Check sheet for the modelled part. Datum: model origin and axes. Units: mm. Face numbers are marked on the shaded views. A direction names the side the tool comes from. Give positions to 0.01 mm unless a question says otherwise; leave off trailing zeros. Loops run counter-clockwise (first coordinate to the right, second up) from the corner with the lowest first, then second, coordinate; pieces in that order, holes last. Notation, with made-up numbers: M 89.25,68 L 142.25,68 A24 cw 142.25,88 Z; hole C 67.25,-0.75 d3. An arc over 180 degrees is marked long. One line per question, with ' | ' between items. Start each with the question number.
from build123d import *

# Parameters (mm, degrees)
SKETCH3_W          = 10.3
SKETCH3_H          = 10.3
CUT_EXTRUDE1_DEPTH = 10.4
SKETCH4_R          = 2.15
CUT_EXTRUDE2_DEPTH = 16.780339887
CUT_EXTRUDE3_START = -10
SKETCH5_R          = 4.5
CUT_EXTRUDE3_DEPTH = 6.62545693
CHAMFER1_SIZE      = 0.5
CHAMFER1_SIZE2     = 1.37373871


with BuildPart() as part:
    # Sketch2 → Revolve1 (revolve)
    with BuildSketch(Plane(origin=(0, 0, 0), x_dir=(1, 0, 0), z_dir=(0, 1, 0))):
        with BuildLine():
            Line((0, 15), (0, -11.180339887))
            Line((0, -11.180339887), (10, -11.180339887))
            ThreePointArc((10, -11.180339887), (14.012585384, 5.352331347), (0, 15))
        make_face()
    revolve(axis=Axis((0, 0, 15), (0, 0, -1)))

    # Sketch3 → Cut-Extrude1 (cut)
    with BuildSketch(Plane.XY.offset(11.180339887)):
        Rectangle(SKETCH3_W, SKETCH3_H)
    extrude(amount=-CUT_EXTRUDE1_DEPTH, mode=Mode.SUBTRACT)

    # Sketch4 → Cut-Extrude2 (cut, through all)
    with BuildSketch(Plane.XY.offset(0.780339887)):
        Circle(SKETCH4_R)
    extrude(amount=-CUT_EXTRUDE2_DEPTH, mode=Mode.SUBTRACT)

    # Sketch5 → Cut-Extrude3 (cut, through all)
    with BuildSketch(Plane.XY.offset(0.780339887).offset(CUT_EXTRUDE3_START)):
        Circle(SKETCH5_R)
    extrude(amount=-CUT_EXTRUDE3_DEPTH, mode=Mode.SUBTRACT)

    # Chamfer1
    chamfer1_edges = [part.edges().sort_by_distance(p)[0] for p in [
        (5.15, 0, 11.180339887),
        (0, 5.15, 11.180339887),
        (-5.15, 0, 11.180339887),
        (0, -5.15, 11.180339887),
    ]]
    chamfer1_side = [part.faces().sort_by_distance(p)[0] for p in [
        (-9.717157288, 0, 11.180339887),
    ]]
    chamfer(chamfer1_edges, length=CHAMFER1_SIZE, length2=CHAMFER1_SIZE2, reference=chamfer1_side[0])


solid = part.part
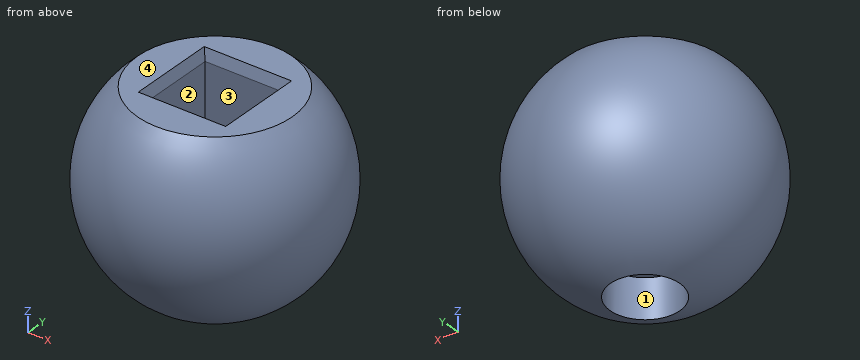
Q1. Material ranges on probe 1 along X at (y, z) = (-0.5, -3.75); probe 2 along Z at (x, y) = (-2.75, -0.25); probe 3 along X at (y, z) = (0, -10.75), recorded low to high. Write a range as from..to.
Q2. Access from +Z, -Z, +X, -X, +Y, -Y to the whole of each face (thin tool, end or side, straight path). Record for the marked faces 1 and 2.
Q3. Cross-section at C-C (z = 8.25). Record the cut outline in (x, y), and give its area (3 significant figures).
Q4. Depth check by flat-ended pin: P1, Ø3, axis at x = 7.5, z = -1.5, coming from the -Y side; P2, Ø4.5, axis at x = 0.5, z = 4.5, coming from the +Y side; P3, Ø11.5, axis at x = -2.5, y = 1, coming from the +Z side; P4, Ø4.5, axis at x = 0, z = 7, coming from the -Y side. Enter the tip coordinate at first touch or a pass-through.
Q5. Cross-section at D-D (z = -8). Record the cut outline in (x, y).
Q6. Cross-section at A-A (x = 0). Record the cut outline in (y, z), and give its area (3 significant figures).
Q7. Draft check along Y on the marked faces 3 and 4. Enter one of: released by +Y, released by -Y, zero draft, split by the parting line, or undercut.
Solved:
1) probe 1: x = -14.52..-2.09, 2.09..14.52 | probe 2: z = -9.22..0.78 | probe 3: x = -10.46..-4.5, 4.5..10.46
2) face 1: -Z | face 2: +Z
3) outline: C 0,0 d25.05; hole M -5.15,-5.15 L 5.15,-5.15 L 5.15,5.15 L -5.15,5.15 Z | area: 387 mm²
4) P1: stops at y = -13.68 | P2: stops at y = 14.83 | P3: stops at z = 11.18 | P4: stops at y = -14.23
5) outline: C 0,0 d25.38; hole C 0,0 d4.3
6) outline: M -10,11.18 A15 ccw -4.5,-14.31 L -4.5,-9.22 L -2.15,-9.22 L -2.15,0.78 L -5.15,0.78 L -5.15,9.81 L -5.65,11.18 Z; M 2.15,-9.22 L 4.5,-9.22 L 4.5,-14.31 A15 ccw 10,11.18 L 5.65,11.18 L 5.15,9.81 L 5.15,0.78 L 2.15,0.78 Z | area: 454 mm²
7) face 3: undercut | face 4: zero draft
